Read the model definition and answer for the solid it produces. Units are mm, in the model's axes. Face numbers are marked on the shaded views. Round coordinates to 2 decimals unless told otherwise and drop trailing zeros. Order: outer loops, then holes, each group sorted by start corner. A loop starts at its lowest first (then second) coordinate and runs counter-clockwise, first axis right, second up. Notation, with made-up numbers: (10.25, 6.5) - (34.25, 6.5) arc R15 ccw to (34.25, 20.5) - close; hole circle Ø1 at (52.25, -16). An arc over 180 degrees is marked (long way). Put each result on its own line as item: value. Start each with the question number.
Q1. For a pull along Z with two mould halves and no side action, classify the marked faces 1, 2, 3 and 4 as pulls with the +Z half, pulls with the -Z half, needs draft (parallel to the pull), parting line crosses it, or undercut.
Q2. Section B-B on z = 0 is taken. State how many separate pieces and enclosed holes the cut face has, then the cut area to 3 significant figures.
Q3. Find the intervals of material crossed by line 1 along Z through (x, y) = (3.25, 38); line 2 along X through (y, z) = (2, -0.5); line 3 along Y through (x, z) = (40, -4), in increasing order. Write a range as from..to.
Q4. Section A-A on z = 4.25 is taken. Give the vertices of the cut face in (x, y), then the cut area to 3 significant figures.
Q5. Section C-C on y = 45 is taken. Give the vertices of the cut face in (x, z).
Q6. Each of these flat-tipped pins is pushed along its axis until it touches: pin 1 Ø2 at (y, z) = (7, 2) entering from +X; pin 2 Ø1 at (y, z) = (8.5, -7.5) entering from +X; pin 3 Ø8 at (x, z) = (12, 0) entering from +Y; pin 4 Ø6.5 at (x, z) = (38, 0) entering from -Y. Where does it stop, or does it pass through?
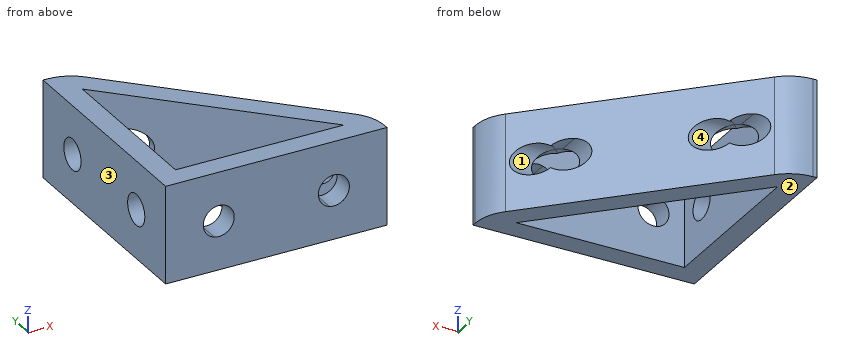
from build123d import *

# Parameters (mm, degrees)
BOSS_EXTRUDE1_DEPTH = 11
FILLET1_R           = 10
FILLET2_R           = 10
SKETCH2_R           = 3.5
CUT_EXTRUDE2_DEPTH  = 72.561162651
CUT_EXTRUDE3_DEPTH  = 46.5


# Read off the part's stored shape, not the designer's step: Cut-Extrude3
with BuildPart() as part:
    # Sketch1 → Boss-Extrude1 (new, symmetric)
    with BuildSketch(Plane.XY):
        Polygon((0, 50), (0, 0), (50, 0), (50, 5), (5, 50), align=None)
        Polygon((43, 5), (5, 5), (5, 43), align=None, mode=Mode.SUBTRACT)
    extrude(amount=BOSS_EXTRUDE1_DEPTH, both=True)

    # Fillet1
    fillet1_edges = [part.edges().sort_by_distance(p)[0] for p in [
        (5, 50, 0),
    ]]
    fillet(fillet1_edges, radius=FILLET1_R)

    # Fillet2
    fillet2_edges = [part.edges().sort_by_distance(p)[0] for p in [
        (50, 5, 0),
    ]]
    fillet(fillet2_edges, radius=FILLET2_R)

    # Sketch2 → Cut-Extrude2 (cut, through all)
    with BuildSketch(Plane.ZY):
        with Locations(Location((0, 38, 0), (0, 0, 270))):
            Circle(SKETCH2_R)
        with Locations(Location((0, 12, 0), (0, 0, 270))):
            Circle(SKETCH2_R)
    extrude(amount=-CUT_EXTRUDE2_DEPTH, mode=Mode.SUBTRACT)

    # Cut-Extrude3 outline → Cut-Extrude3 (cut)
    with BuildSketch(Plane(origin=(0, 0, 0), x_dir=(1, 0, 0), z_dir=(0, 1, 0))):
        with BuildLine():
            ThreePointArc((11, -3.354101966), (15.5, 0), (11, 3.354101966))
            ThreePointArc((11, 3.354101966), (8.5, 0), (11, -3.354101966))
        make_face()
        with BuildLine():
            ThreePointArc((37, -3.354101966), (41.5, 0), (37, 3.354101966))
            ThreePointArc((37, 3.354101966), (34.5, 0), (37, -3.354101966))
        make_face()
    extrude(amount=CUT_EXTRUDE3_DEPTH, mode=Mode.SUBTRACT)


solid = part.part
Findings:
1. face 1: undercut
1. face 2: pulls with the -Z half
1. face 3: needs draft
1. face 4: undercut
2. separate pieces: 6
2. enclosed holes: 0
2. area: 494 mm2
3. line 1: -11..-3.5, 3.5..11
3. line 2: 0..8.54, 15.46..34.54, 41.46..49.93
3. line 3: 0..5, 8..15
4. outline: (0, 0) - (50, 0) - (50, 0.86) arc R10 ccw to (47.07, 7.93) - (7.93, 47.07) arc R10 ccw to (0.86, 50) - (0, 50) - close; hole (5, 5) - (43, 5) - (5, 43) - close
4. area: 761 mm2
5. outline: (0, -11) - (10, -11) - (10, -2.87) arc R3.5 cw to (10, 2.87) - (10, 11) - (0, 11) - close
6. pin 1: x = 48.58
6. pin 2: x = 47
6. pin 3: y = 47
6. pin 4: through
